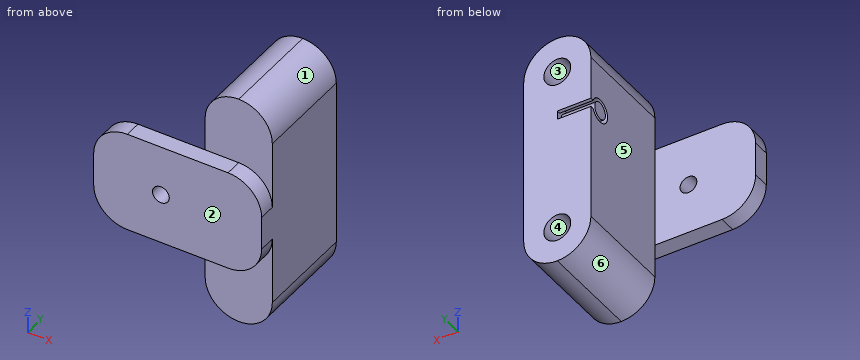
from build123d import *

# Parameters (mm, degrees)
SKETCH2_W           = 20
SKETCH2_H           = 70
BOSS_EXTRUDE1_DEPTH = 30
SKETCH3_R           = 4
CUT_EXTRUDE1_DEPTH  = 20
SKETCH4_R           = 2.5
CUT_EXTRUDE2_DEPTH  = 10
FILLET1_R           = 10
SKETCH6_W           = 50
SKETCH6_H           = 30
BOSS_EXTRUDE3_DEPTH = 5
SKETCH7_R           = 2.5
CUT_EXTRUDE3_DEPTH  = 10
FILLET3_R           = 10


with BuildPart() as part:
    # Sketch2 → Boss-Extrude1 (new body)
    with BuildSketch(Plane(origin=(0, 0, 0), x_dir=(1, 0, 0), z_dir=(0, 1, 0))):
        with Locations((6.47761194, -5.23880597)):
            Rectangle(SKETCH2_W, SKETCH2_H)
    extrude(amount=BOSS_EXTRUDE1_DEPTH)

    # Sketch3 → Cut-Extrude1 (cut)
    with BuildSketch(Plane(origin=(0, 30, 0), x_dir=(1, 0, 0), z_dir=(0, 1, 0))):
        with Locations(Location((6.47761194, 19.26119403, 0), (0, 0, 270))):
            Circle(SKETCH3_R)
        with Locations(Location((6.47761194, -29.73880597, 0), (0, 0, 270))):
            Circle(SKETCH3_R)
    extrude(amount=-CUT_EXTRUDE1_DEPTH, mode=Mode.SUBTRACT)

    # Sketch4 → Cut-Extrude2 (cut)
    with BuildSketch(Plane.ZY.offset(3.52238806)):
        with BuildLine():
            Line((17.415034126, 30.126407987), (14.795699792, 30.126407987))
            Line((14.795699792, 30.126407987), (14.949961333, 28.969446425))
            ThreePointArc((14.949961333, 28.969446425), (16.17927412, 22.186618473), (17.347611009, 28.980215007))
            Line((17.347611009, 28.980215007), (17.415034126, 30.126407987))
        make_face()
        with Locations((16.163554702, 25.686583173)):
            Circle(SKETCH4_R, mode=Mode.SUBTRACT)
    extrude(amount=-CUT_EXTRUDE2_DEPTH, mode=Mode.SUBTRACT)

    # Fillet1
    fillet1_edges = [part.edges().sort_by_distance(p)[0] for p in [
        (-3.52238806, 15, -29.76119403),
        (16.47761194, 15, -29.76119403),
        (16.47761194, 15, 40.23880597),
        (-3.52238806, 15, 40.23880597),
    ]]
    fillet(fillet1_edges, radius=FILLET1_R - 0.0001)  # a hair under: the kernel refuses the full size

    # Sketch6 → Boss-Extrude3 (add)
    with BuildSketch(Plane.XZ):
        with Locations((-8.52238806, 5.23880597)):
            Rectangle(SKETCH6_W, SKETCH6_H)
    extrude(amount=BOSS_EXTRUDE3_DEPTH)

    # Sketch7 → Cut-Extrude3 (cut)
    with BuildSketch(Plane.XZ.offset(5)):
        with Locations(Location((-13.52238806, 5.23880597, 0), (0, 0, 270))):
            Circle(SKETCH7_R)
    extrude(amount=-CUT_EXTRUDE3_DEPTH, mode=Mode.SUBTRACT)

    # Fillet3
    fillet3_edges = [part.edges().sort_by_distance(p)[0] for p in [
        (-33.52238806, -2.5, 20.23880597),
        (-33.52238806, -2.5, -9.76119403),
        (16.47761194, -2.5, -9.76119403),
        (16.47761194, -2.5, 20.23880597),
    ]]
    fillet(fillet3_edges, radius=FILLET3_R)


solid = part.part
Here's how the part is built. I have some questions about the finished solid (model axes, mm). Face numbers are marked on the shaded views. A direction names the side the tool comes from. Give positions to 0.01 mm unless a question says otherwise; leave off trailing zeros. Order: outer loops, then holes, each group sorted by start corner. A loop starts at its lowest first (then second) coordinate and runs counter-clockwise, first axis right, second up. Notation, with made-up numbers: (-24.75, 10.5) -> (-10.75, 10.5) arc R23 ccw to (-10.75, 21.5) -> close; hole circle Ø2 at (-35.75, -6). An arc over 180 degrees is marked (long way). One line per item, written item: value. Start each with the question number.
1. Will these pins go through, and if not, where does the flat tip stop? pin 1 Ø24 at (x, z) = (-20.5, 4) entering from +Y; pin 2 Ø7 at (x, z) = (6.48, 29.74) entering from -Y; pin 3 Ø2 at (y, z) = (28, 16) entering from -X.
2. Imagine slicing it at B-B, the plane z = 5.5. List the corners of the cut face in (x, y) for me.
3. Imagine slicing it at D-D, the plane x = -2. List the corners of the cut face in (y, z) for me.
4. I need wall thicknesses on probe 1 along X at (y, z) = (6.5, 6); probe 2 along X at (y, z) = (28.5, 17); probe 3 along Z at (x, y) = (6, 6). Which ranges of each line are inside material? Lowest first, please. Write a range as from..to.
5. For the marked faces 5 and 6, which set-ups out of +Z, -Z, +X, -X, +Y, -Y let a thin tool reach every point of the face, with its end or its side?
6. Imagine slicing it at A-A, the plane y = 13. Count the separate pieces of the cut face and the enclosed holes in it, plus the area to 3 significant figures.
7. We'd pull the mould along Z, two halves only. Please class the marked faces 1, 2, 3 and 4: released by +Z, released by -Z, zero draft, split by the parting line, or undercut.
Values follow:
1. pin 1: stops at y = 0
1. pin 2: stops at y = 0
1. pin 3: stops at x = -3.52
2. outline: (-33.52, -5) -> (-16.01, -5) -> (-16.01, 0) -> (-33.52, 0) -> close; (-11.04, -5) -> (16.48, -5) -> (16.48, 30) -> (-3.52, 30) -> (-3.52, 0) -> (-11.04, 0) -> close
3. outline: (-5, -9.76) -> (0, -9.76) -> (0, -25.07) -> (30, -25.07) -> (30, 14.81) -> (28.97, 14.95) arc R3.5 cw (long way) to (28.98, 17.35) -> (30, 17.41) -> (30, 35.54) -> (0, 35.54) -> (0, 20.24) -> (-5, 20.24) -> close; circle Ø5 at (25.69, 16.16)
4. probe 1: x = -3.52..16.48
4. probe 2: x = 6.48..16.48
4. probe 3: z = -29.75..40.23
5. face 5: +Z, -Z, -X, +Y
5. face 6: -Z, -X, +Y, -Y
6. separate pieces: 1
6. enclosed holes: 2
6. area: 1,210 mm2
7. face 1: released by +Z
7. face 2: zero draft
7. face 3: undercut
7. face 4: undercut
